from build123d import *

# Parameters (mm, degrees)
SKETCH1_W                    = 30
SKETCH1_H                    = 55
SKETCH1_W_2                  = 20
SKETCH1_H_2                  = 40
SERVO_MOUNT_DEPTH            = 3
F_4_0_4_DIAMETER_HOLE1_D     = 4
F_4_0_4_DIAMETER_HOLE1_DEPTH = 4
F_4_0_4_DIAMETER_HOLE1_TIP   = 1.201721238
SKETCH4_W                    = 10
SKETCH4_H                    = 55
AXLE_MOUNT_BASE_DEPTH        = 3
AXLE_START                   = 3
SKETCH4_3_R                  = 0.975
AXLE_MOUNT_DEPTH             = 3


with BuildPart() as part:
    # Sketch1 → Servo Mount (new body)
    with BuildSketch(Plane.XY):
        with Locations((0, 20)):
            Rectangle(SKETCH1_W, SKETCH1_H)
        with Locations((0, 20)):
            Rectangle(SKETCH1_W_2, SKETCH1_H_2, mode=Mode.SUBTRACT)
    extrude(amount=SERVO_MOUNT_DEPTH)

    # Ø4.0 (4) Diameter Hole1
    with Locations(Plane.XY.offset(3)):
        with Locations((-6.7, 44.2), (-6.7, -4.2), (6.7, 44.2), (6.7, -4.2)):
            Hole(F_4_0_4_DIAMETER_HOLE1_D / 2, depth=F_4_0_4_DIAMETER_HOLE1_DEPTH)
            with Locations((0, 0, -(F_4_0_4_DIAMETER_HOLE1_DEPTH + F_4_0_4_DIAMETER_HOLE1_TIP / 2))):  # 118° drill point
                Cone(0, F_4_0_4_DIAMETER_HOLE1_D / 2, F_4_0_4_DIAMETER_HOLE1_TIP, mode=Mode.SUBTRACT)

    # Sketch4 → Axle Mount Base (add)
    with BuildSketch(Plane(origin=(15, 0, 0), x_dir=(0, 0, -1), z_dir=(1, 0, 0))):
        with Locations((-5, 20)):
            Rectangle(SKETCH4_W, SKETCH4_H)
    extrude(amount=AXLE_MOUNT_BASE_DEPTH)

    # Sketch4<3> → Axle Mount (add)
    with BuildSketch(Plane(origin=(15, 0, 0), x_dir=(0, 0, -1), z_dir=(1, 0, 0)).offset(AXLE_START)):
        with BuildLine():
            Line((-3, 17.865608986), (-3, 16.622778509))
            ThreePointArc((-3, 16.622778509), (-1.590042156, 18.056340436), (-1.075, 20))
            ThreePointArc((-1.075, 20), (-1.590042156, 21.943659564), (-3, 23.377221491))
            Line((-3, 23.377221491), (-3, 22.134391014))
            ThreePointArc((-3, 22.134391014), (-2.3161944, 21.163104681), (-2.075, 20))
            ThreePointArc((-2.075, 20), (-2.3161944, 18.836895319), (-3, 17.865608986))
        make_face()
        with BuildLine():
            ThreePointArc((-3, 23.377221491), (-8.925, 20), (-3, 16.622778509))
            Line((-3, 16.622778509), (-3, 17.865608986))
            ThreePointArc((-3, 17.865608986), (-7.925, 20), (-3, 22.134391014))
            Line((-3, 22.134391014), (-3, 23.377221491))
        make_face()
        with Locations(Location((-5, 20, 0), (0, 0, 180))):
            Circle(SKETCH4_3_R)
    extrude(amount=AXLE_MOUNT_DEPTH)


solid = part.part
Read the model definition and answer for the solid it produces. Units are mm, in the model's axes. A direction names the side the tool comes from. Round coordinates to 2 decimals unless told otherwise and drop trailing zeros. Write each loop counter-clockwise with the first axis right and the second up, starting at its lowest first coordinate (ties: lowest second). Pieces come first, ordered by that corner, then holes.
1. The part is cut by section C-C, the plane x = 0. Determine the outline of the cut face in (y, z), then the cut area to 3 significant figures.
2. Straight lines are drawn through the part: L1, parallel to Y at x = 6.7, z = 2; L2, parallel to X at y = 18, z = 1; L3, parallel to Y at x = 8.5, z = 2.25. For each, find the intervals that lie inside material, in ascending order.
3. Determine the mould class of faces 1 (the face through (16, 20, 10)), 2 (the face through (21, 23, 6)), 3 (the face through (10, 20, 1)), 4 (the face through (7.134, -6.152, 1.479)) for opening direction X: pulls with the +X half, pulls with the -X half, needs draft (parallel to the pull), parting line crosses it, or undercut.
4. The part is cut by section B-B, the plane x = -6.7. Determine the outline of the cut face in (y, z), then the cut area to 3 significant figures.
5. Given pin 1 Ø3 at (y, z) = (7, 7) entering from +X; pin 2 Ø2 at (y, z) = (26, 5) entering from -X, each flat-ended and moving along its own axis, determine where each tip first touches the part or whether it passes through.
6. The part is cut by section A-A, the plane y = 3. Determine the outline of the cut face in (x, z), then the cut area to 3 significant figures.
7. The part is cut by section D-D, the plane y = -4.2. Determine the outline of the cut face in (x, z).
8. Which of the six approach directions +Z, -Z, +X, -X, +Y, -Y give full straight-line access (tool end or side, diameter ignored) to faces 5 (the face through (15, 20, 7)), 6 (the face through (-15, 20, 1)), 7 (the face through (4.9, -7.5, 2.8)), 8 (the face through (18, 21, 6)), 9 (the face through (0, 40, 1))?
Values:
1. outline: (-7.5, 0) - (0, 0) - (0, 3) - (-7.5, 3) - close; (40, 0) - (47.5, 0) - (47.5, 3) - (40, 3) - close
1. area: 45.0 mm2
2. L1: y = -7.5 to -6.2, -2.2 to 0, 40 to 42.2, 46.2 to 47.5
2. L2: x = -15 to -10, 10 to 18
2. L3: y = -7.5 to -5.07, -3.33 to 0, 40 to 43.33, 45.07 to 47.5
3. face 1: needs draft
3. face 2: pulls with the +X half
3. face 3: undercut
3. face 4: undercut
4. outline: (-7.5, 0) - (-6.2, 0) - (-6.2, 3) - (-7.5, 3) - close; (-2.2, 0) - (0, 0) - (0, 3) - (-2.2, 3) - close; (40, 0) - (42.2, 0) - (42.2, 3) - (40, 3) - close; (46.2, 0) - (47.5, 0) - (47.5, 3) - (46.2, 3) - close
4. area: 21.0 mm2
5. pin 1: stops at x = 18
5. pin 2: stops at x = 15
6. outline: (-15, 0) - (-10, 0) - (-10, 3) - (-15, 3) - close; (10, 0) - (18, 0) - (18, 10) - (15, 10) - (15, 3) - (10, 3) - close
6. area: 60.0 mm2
7. outline: (-15, 0) - (-8.7, 0) - (-8.7, 3) - (-15, 3) - close; (-4.7, 0) - (4.7, 0) - (4.7, 3) - (-4.7, 3) - close; (8.7, 0) - (18, 0) - (18, 10) - (15, 10) - (15, 3) - (8.7, 3) - close
8. face 5: +Z, -X, +Y, -Y
8. face 6: +Z, -Z, -X, +Y, -Y
8. face 7: +Z, -Z, +X, -X, -Y
8. face 8: +X
8. face 9: +Z, -Z
